The listing builds one solid part. Answer for the finished solid, in the listing's coordinates (mm). A direction names the side the tool comes from. Give positions to 0.01 mm unless a question says otherwise; leave off trailing zeros. Write each loop counter-clockwise with the first axis right and the second up, starting at its lowest first coordinate (ties: lowest second). Pieces come first, ordered by that corner, then holes. Notation, with made-up numbers: (83.25, 42) - (126.25, 42) arc R34 ccw to (126.25, 75) - close; hole circle Ø3 at (2.25, 15). An arc over 180 degrees is marked (long way). Write each question's results on one line, items separated by ' | '. Start each with the question number.
Q1. Find the intervals of material crossed by probe 1 along Z at (x, y) = (-76, 3.6); probe 2 along X at (y, z) = (2, -57); probe 3 along X at (y, z) = (7.75, -17.5), in increasing order.
Q2. Section A-A (z = -32.5) is taken. Determine the outline of the cut face in (x, y), plus the area to 4 significant figures.
Q3. For a pull along Z with two mould halves and no side action, classify faces 1 (the face through (-101.15, 2.54, -70.49)), 2 (the face through (17, 6, -32)), 3 (the face through (-17, 10, -50)) as pulls with the +Z half, pulls with the -Z half, needs draft (parallel to the pull), parting line crosses it, or undercut.
Q4. For faces 4 (the face through (29, 3, -57)), 5 (the face through (20, 6.5, -32)), 6 (the face through (-40.476, 3, 0)), 7 (the face through (-22, 3, 60.028)), determine the directions among +Z, -Z, +X, -X, +Y, -Y from which every point of the face is accessible in a straight line to the end or side of a thin tool.
Q5. Section B-B (y = 1.5) is taken. State how many separate pieces and enclosed holes the cut face has, plus the area to 3 significant figures.
Q6. Flat-ended cylindrical pins translate along their axes: pin 1 Ø2 at (x, y) = (-18.5, 3.5) entering from +Z; pin 2 Ø6 at (x, y) = (-51.5, 8.5) entering from +Z; pin 3 Ø1.5 at (y, z) = (1.5, -66.5) entering from +X; pin 4 Ø3.5 at (x, z) = (-47.39, 50.03) entering from +Y. Find the tip coordinate at first contact, or state that the pin passes through.
```python
from build123d import *

# Parameters (mm, degrees)
SKETCH1_W            = 208
SKETCH1_H            = 147
BOSS_EXTRUDE1_DEPTH  = 5
CUT_EXTRUDE2_DEPTH   = 128.449009412
MIRROR2_COPY_1_DEPTH = 128.449009412
FILLET1_R            = 10
CUT_EXTRUDE3_DEPTH   = 128.449009412
SKETCH5_R            = 1.6
CUT_EXTRUDE4_DEPTH   = 10
SKETCH8_R            = 1.6
CUT_EXTRUDE5_DEPTH   = 10
SKETCH9_W            = 43
SKETCH9_H            = 43
SKETCH9_W_2          = 33
SKETCH9_H_2          = 33
BOSS_EXTRUDE3_DEPTH  = 5
SKETCH10_W           = 27
SKETCH10_H           = 3.5
CUT_EXTRUDE6_DEPTH   = 62
SKETCH11_W           = 27
SKETCH11_H           = 3.5
CUT_EXTRUDE7_DEPTH   = 62
FILLET4_R            = 3.5
SKETCH12_R           = 1.6
CUT_EXTRUDE8_DEPTH   = 62
FILLET5_R            = 3.5
FILLET6_R            = 2
SKETCH14_W           = 15
SKETCH14_H           = 13.472377551
CUT_EXTRUDE10_DEPTH  = 10


with BuildPart() as part:
    # Sketch1 → Boss-Extrude1 (new body)
    with BuildSketch(Plane(origin=(0, 0, 0), x_dir=(1, 0, 0), z_dir=(0, 1, 0))):
        Rectangle(SKETCH1_W, SKETCH1_H)
    extrude(amount=BOSS_EXTRUDE1_DEPTH)

    # Sketch2 → Cut-Extrude2 (cut, through all)
    with BuildSketch(Plane(origin=(0, 5, 0), x_dir=(1, 0, 0), z_dir=(0, 1, 0))):
        with BuildLine():
            Line((-89, 80.027622449), (-89, 60.027622449))
            Line((-89, 60.027622449), (-44, 60.027622449))
            Line((-44, 60.027622449), (-44, 55.027622449))
            Line((-44, 55.027622449), (-29, 55.027622449))
            Line((-29, 55.027622449), (-29, 60.027622449))
            Line((-29, 60.027622449), (-14, 60.027622449))
            ThreePointArc((-14, 60.027622449), (-6.928932188, 60.530147766), (0, 62.027622449))
            Line((0, 62.027622449), (0, 82.027622449))
            Line((0, 82.027622449), (-89, 82.027622449))
            Line((-89, 82.027622449), (-89, 80.027622449))
        make_face()
    cut_extrude2 = extrude(amount=-CUT_EXTRUDE2_DEPTH, mode=Mode.SUBTRACT)

    # Mirror1: Cut-Extrude2 across plane
    add(cut_extrude2.mirror(Plane.XY), mode=Mode.SUBTRACT)

    # Mirror2: Cut-Extrude2 across plane
    add(cut_extrude2.mirror(Plane(origin=(0, 0, 0), x_dir=(0, 0, 1), z_dir=(1, 0, 0))), mode=Mode.SUBTRACT)

    # Mirror2 copy 1 sketch → Mirror2 copy 1 (cut, through all)
    with BuildSketch(Plane(origin=(0, 5, 0), x_dir=(-1, 0, 0), z_dir=(0, 1, 0))):
        with BuildLine():
            Line((-89, 80.027622449), (-89, 60.027622449))
            Line((-89, 60.027622449), (-44, 60.027622449))
            Line((-44, 60.027622449), (-44, 55.027622449))
            Line((-44, 55.027622449), (-29, 55.027622449))
            Line((-29, 55.027622449), (-29, 60.027622449))
            Line((-29, 60.027622449), (-14, 60.027622449))
            ThreePointArc((-14, 60.027622449), (-6.928932188, 60.530147766), (0, 62.027622449))
            Line((0, 62.027622449), (0, 82.027622449))
            Line((0, 82.027622449), (-89, 82.027622449))
            Line((-89, 82.027622449), (-89, 80.027622449))
        make_face()
    extrude(amount=-MIRROR2_COPY_1_DEPTH, mode=Mode.SUBTRACT)

    # Fillet1
    fillet1_edges = [part.edges().sort_by_distance(p)[0] for p in [
        (-104, 2.5, -73.5),
        (104, 2.5, -73.5),
        (104, 2.5, 73.5),
        (-104, 2.5, 73.5),
    ]]
    fillet(fillet1_edges, radius=FILLET1_R)

    # Sketch3 → Cut-Extrude3 (cut, through all)
    with BuildSketch(Plane(origin=(0, 5, 0), x_dir=(1, 0, 0), z_dir=(0, 1, 0))):
        with BuildLine():
            Line((-56.39463696, -4.457125787), (-56.39463696, -11.538322368))
            ThreePointArc((-56.39463696, -11.538322368), (-56.101743741, -12.245429149), (-55.39463696, -12.538322368))
            Line((-55.39463696, -12.538322368), (-51.39463696, -12.538322368))
            ThreePointArc((-51.39463696, -12.538322368), (-50.687530178, -12.245429149), (-50.39463696, -11.538322368))
            Line((-50.39463696, -11.538322368), (-50.39463696, -4.457125787))
            ThreePointArc((-50.39463696, -4.457125787), (-50.101743741, -3.750019006), (-49.39463696, -3.457125787))
            Line((-49.39463696, -3.457125787), (-41.475833541, -3.457125787))
            ThreePointArc((-41.475833541, -3.457125787), (-40.76872676, -3.164232568), (-40.475833541, -2.457125787))
            Line((-40.475833541, -2.457125787), (-40.475833541, 1.542874213))
            ThreePointArc((-40.475833541, 1.542874213), (-40.76872676, 2.249980994), (-41.475833541, 2.542874213))
            Line((-41.475833541, 2.542874213), (-49.39463696, 2.542874213))
            ThreePointArc((-49.39463696, 2.542874213), (-50.101743741, 2.835767432), (-50.39463696, 3.542874213))
            Line((-50.39463696, 3.542874213), (-50.39463696, 11.461677632))
            ThreePointArc((-50.39463696, 11.461677632), (-50.687530178, 12.168784413), (-51.39463696, 12.461677632))
            Line((-51.39463696, 12.461677632), (-55.39463696, 12.461677632))
            ThreePointArc((-55.39463696, 12.461677632), (-56.101743741, 12.168784413), (-56.39463696, 11.461677632))
            Line((-56.39463696, 11.461677632), (-56.39463696, 3.542874213))
            ThreePointArc((-56.39463696, 3.542874213), (-56.687530178, 2.835767432), (-57.39463696, 2.542874213))
            Line((-57.39463696, 2.542874213), (-64.475833541, 2.542874213))
            ThreePointArc((-64.475833541, 2.542874213), (-65.182940322, 2.249980994), (-65.475833541, 1.542874213))
            Line((-65.475833541, 1.542874213), (-65.475833541, -2.457125787))
            ThreePointArc((-65.475833541, -2.457125787), (-65.182940322, -3.164232568), (-64.475833541, -3.457125787))
            Line((-64.475833541, -3.457125787), (-57.39463696, -3.457125787))
            ThreePointArc((-57.39463696, -3.457125787), (-56.687530178, -3.750019006), (-56.39463696, -4.457125787))
        make_face()
    extrude(amount=-CUT_EXTRUDE3_DEPTH, mode=Mode.SUBTRACT)

    # Sketch5 → Cut-Extrude4 (cut)
    with BuildSketch(Plane(origin=(0, 5, 0), x_dir=(1, 0, 0), z_dir=(0, 1, 0))):
        with Locations(Location((-96, 20.039754171, 0), (0, 0, 270))):
            Circle(SKETCH5_R)
        with Locations(Location((-76, 20.039754171, 0), (0, 0, 270))):
            Circle(SKETCH5_R)
        with Locations(Location((-76, 0.039754171, 0), (0, 0, 270))):
            Circle(SKETCH5_R)
        with Locations(Location((-96, 0.039754171, 0), (0, 0, 270))):
            Circle(SKETCH5_R)
    extrude(amount=-CUT_EXTRUDE4_DEPTH, mode=Mode.SUBTRACT)

    # Sketch8 → Cut-Extrude5 (cut)
    with BuildSketch(Plane(origin=(0, 5, 0), x_dir=(1, 0, 0), z_dir=(0, 1, 0))):
        with Locations(Location((-59.39463696, -50.027622449, 0), (0, 0, 270))):
            Circle(SKETCH8_R)
        with Locations(Location((-47.39463696, -50.027622449, 0), (0, 0, 270))):
            Circle(SKETCH8_R)
        with Locations(Location((-47.39463696, -38.027622449, 0), (0, 0, 270))):
            Circle(SKETCH8_R)
        with Locations(Location((-59.39463696, -38.027622449, 0), (0, 0, 270))):
            Circle(SKETCH8_R)
        with Locations(Location((-59.39463696, 50.027622449, 0), (0, 0, 90))):
            Circle(SKETCH8_R)
        with Locations(Location((-47.39463696, 50.027622449, 0), (0, 0, 90))):
            Circle(SKETCH8_R)
        with Locations(Location((-47.39463696, 38.027622449, 0), (0, 0, 90))):
            Circle(SKETCH8_R)
        with Locations(Location((-59.39463696, 38.027622449, 0), (0, 0, 90))):
            Circle(SKETCH8_R)
        with Locations(Location((59.39463696, 50.027622449, 0), (0, 0, 270))):
            Circle(SKETCH8_R)
        with Locations(Location((47.39463696, 50.027622449, 0), (0, 0, 270))):
            Circle(SKETCH8_R)
        with Locations(Location((47.39463696, 38.027622449, 0), (0, 0, 270))):
            Circle(SKETCH8_R)
        with Locations(Location((59.39463696, 38.027622449, 0), (0, 0, 270))):
            Circle(SKETCH8_R)
        with Locations(Location((47.39463696, -50.027622449, 0), (0, 0, 90))):
            Circle(SKETCH8_R)
        with Locations(Location((47.39463696, -38.027622449, 0), (0, 0, 90))):
            Circle(SKETCH8_R)
        with Locations(Location((59.39463696, -50.027622449, 0), (0, 0, 90))):
            Circle(SKETCH8_R)
        with Locations(Location((59.39463696, -38.027622449, 0), (0, 0, 90))):
            Circle(SKETCH8_R)
    extrude(amount=-CUT_EXTRUDE5_DEPTH, mode=Mode.SUBTRACT)

    # Sketch9 → Boss-Extrude3 (add)
    with BuildSketch(Plane(origin=(0, 5, 0), x_dir=(1, 0, 0), z_dir=(0, 1, 0))):
        with Locations((0.5, 32.527622449)):
            Rectangle(SKETCH9_W, SKETCH9_H)
        with Locations((0.5, 32.527622449)):
            Rectangle(SKETCH9_W_2, SKETCH9_H_2, mode=Mode.SUBTRACT)
    extrude(amount=BOSS_EXTRUDE3_DEPTH)

    # Sketch10 → Cut-Extrude6 (cut)
    with BuildSketch(Plane.XY.offset(-11.027622449)):
        with Locations((0.5, 8.25)):
            Rectangle(SKETCH10_W, SKETCH10_H)
    extrude(amount=-CUT_EXTRUDE6_DEPTH, mode=Mode.SUBTRACT)

    # Sketch11 → Cut-Extrude7 (cut)
    with BuildSketch(Plane(origin=(22, 0, 0), x_dir=(0, 0, -1), z_dir=(1, 0, 0))):
        with Locations((32.527622449, 8.25)):
            Rectangle(SKETCH11_W, SKETCH11_H)
    extrude(amount=-CUT_EXTRUDE7_DEPTH, mode=Mode.SUBTRACT)

    # Fillet4
    fillet4_edges = [part.edges().sort_by_distance(p)[0] for p in [
        (19.5, 6.5, -19.027622449),
        (19.5, 6.5, -46.027622449),
        (14, 6.5, -51.527622449),
        (-18.5, 6.5, -19.027622449),
        (-18.5, 6.5, -46.027622449),
        (-13, 6.5, -13.527622449),
    ]]
    fillet(fillet4_edges, radius=FILLET4_R - 0.0001)  # a hair under: the kernel refuses the full size

    # Sketch12 → Cut-Extrude8 (cut)
    with BuildSketch(Plane(origin=(0, 10, 0), x_dir=(1, 0, 0), z_dir=(0, 1, 0))):
        with Locations(Location((-18.25, 51.277622449, 0), (0, 0, 270))):
            Circle(SKETCH12_R)
        with Locations(Location((19.25, 51.277622449, 0), (0, 0, 90))):
            Circle(SKETCH12_R)
        with Locations(Location((19.25, 13.777622449, 0), (0, 0, 270))):
            Circle(SKETCH12_R)
        with Locations(Location((-18.25, 13.777622449, 0), (0, 0, 90))):
            Circle(SKETCH12_R)
    extrude(amount=-CUT_EXTRUDE8_DEPTH, mode=Mode.SUBTRACT)

    # Fillet5
    fillet5_edges = [part.edges().sort_by_distance(p)[0] for p in [
        (14, 6.5, -13.527622449),
        (-13, 6.5, -51.527622449),
    ]]
    fillet(fillet5_edges, radius=FILLET5_R - 0.0001)  # a hair under: the kernel refuses the full size

    # Fillet6
    fillet6_edges = [part.edges().sort_by_distance(p)[0] for p in [
        (-21, 7.5, -54.027622449),
        (-21, 7.5, -11.027622449),
        (22, 7.5, -11.027622449),
        (22, 7.5, -54.027622449),
    ]]
    fillet(fillet6_edges, radius=FILLET6_R)

    # Sketch14 → Cut-Extrude10 (cut)
    with BuildSketch(Plane(origin=(0, 5, 0), x_dir=(1, 0, 0), z_dir=(0, 1, 0))):
        with Locations((96.5, 66.763811225)):
            Rectangle(SKETCH14_W, SKETCH14_H)
        with Locations((96.5, -66.763811225)):
            Rectangle(SKETCH14_W, SKETCH14_H)
    extrude(amount=-CUT_EXTRUDE10_DEPTH, mode=Mode.SUBTRACT)


solid = part.part
```
Answers below:
1) probe 1: z = -60.03 to -21.64, -18.44 to -1.64, 1.56 to 60.03 | probe 2: x = -104 to -44, -29 to 29, 44 to 104 | probe 3: x = -21 to -16, 17 to 22
2) outline: (-104, 0) - (104, 0) - (104, 5) - (22, 5) - (22, 6.5) - (17, 6.5) - (17, 5) - (-16, 5) - (-16, 6.5) - (-21, 6.5) - (-21, 5) - (-104, 5) - close | area: 1,055 mm2
3) face 1: pulls with the -Z half | face 2: undercut | face 3: needs draft
4) face 4: -Z, +Y, -Y | face 5: +X, -X, +Y | face 6: +Y, -Y | face 7: +Z, +Y, -Y
5) separate pieces: 1 | enclosed holes: 25 | area: 24,600 mm2
6) pin 1: stops at z = 60.03 | pin 2: passes through | pin 3: stops at x = -89 | pin 4: stops at y = 5
